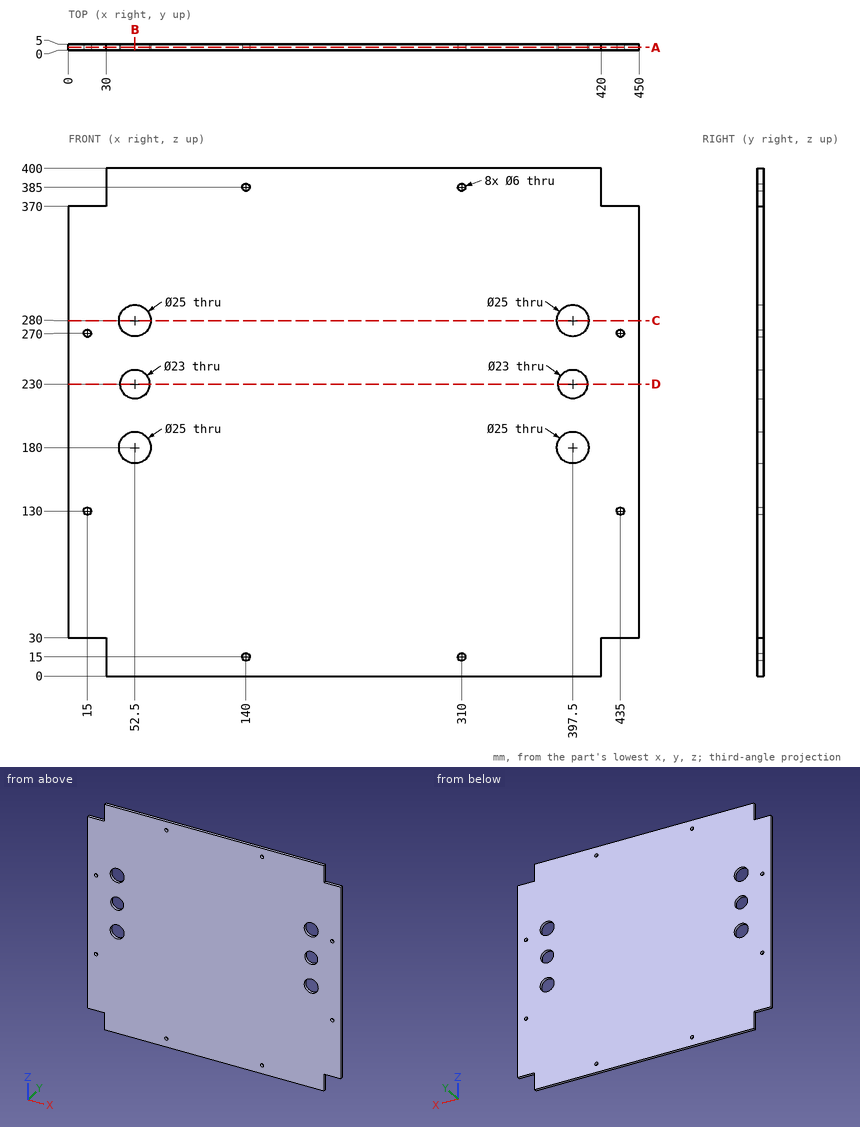
Geometry check sheet. Reference: drawing and pictorial views, mm from the part's lowest x, y, z. Coordinates: 2 decimals unless noted, no trailing zeros. Order: outer loops, then holes, each group sorted by start corner. A loop starts at its lowest first (then second) coordinate and runs counter-clockwise, first axis right, second up. Notation, with made-up numbers: (46, 57.25) -> (68, 57.25) arc R29 ccw to (68, 77.25) -> close; hole circle Ø3 at (69, 62.5). An arc over 180 degrees is marked (long way). Put each result on its own line as item: value. Start each with the question number.
1) Cross-section at A-A (y = 2.25). State how many separate pieces and enclosed holes the cut face has, plus the area to 3 significant figures.
2) Cross-section at C-C (z = 280). Enter the section's corners in (x, y).
3) Cross-section at B-B (x = 52.5). Enter the section's corners in (y, z), plus the area to 4 significant figures.
4) Material ranges on L1, parallel to Z at x = 310, y = 2.25; L2, parallel to Z at x = 397.5, y = 2.55; L3, parallel to X at y = 1.8, z = 180, recorded low to high.
5) Cross-section at D-D (z = 230). Enter the section's corners in (x, y).
6) Go/stop test with a flat-tipped pin: pin 1 (5 mm diameter, centred on x = 435, z = 130, fed in from -Y). Record where the tip stops, or that it passes through.
Geometry check:
1. separate pieces: 1
1. enclosed holes: 14
1. area: 173,000 mm^2
2. outline: (0, 0) -> (40, 0) -> (40, 5) -> (0, 5) -> close; (65, 0) -> (385, 0) -> (385, 5) -> (65, 5) -> close; (410, 0) -> (450, 0) -> (450, 5) -> (410, 5) -> close
3. outline: (0, 0) -> (5, 0) -> (5, 167.5) -> (0, 167.5) -> close; (0, 192.5) -> (5, 192.5) -> (5, 218.5) -> (0, 218.5) -> close; (0, 241.5) -> (5, 241.5) -> (5, 267.5) -> (0, 267.5) -> close; (0, 292.5) -> (5, 292.5) -> (5, 400) -> (0, 400) -> close
3. area: 1,635 mm^2
4. L1: z = 0 to 12, 18 to 382, 388 to 400
4. L2: z = 0 to 167.5, 192.5 to 218.5, 241.5 to 267.5, 292.5 to 400
4. L3: x = 0 to 40, 65 to 385, 410 to 450
5. outline: (0, 0) -> (41, 0) -> (41, 5) -> (0, 5) -> close; (64, 0) -> (386, 0) -> (386, 5) -> (64, 5) -> close; (409, 0) -> (450, 0) -> (450, 5) -> (409, 5) -> close
6. pin 1: passes through
